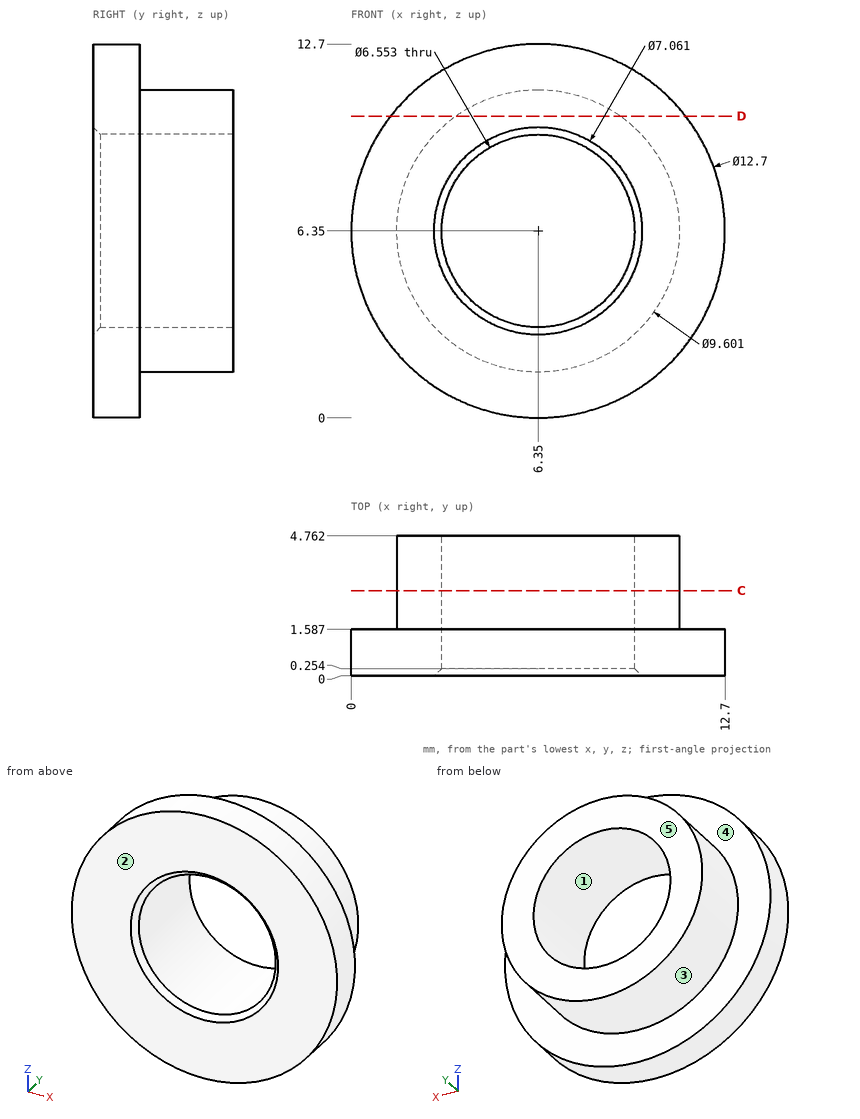
For this review, use the dimensioned drawing (mm, ordinates from the lowest corner) and the shaded views. A direction names the side the tool comes from. Give positions to 0.01 mm unless a question says otherwise; leave off trailing zeros. Loops run counter-clockwise (first coordinate to the right, second up) from the corner with the lowest first, then second, coordinate; pieces in that order, holes last. Notation, with made-up numbers: (67, -39) -> (109, -39) arc R28 cw to (109, -1) -> close; hole circle Ø11 at (0, -34). An arc over 180 degrees is marked (long way). One line per question, with ' | ' between items. Start each with the question number.
(1) Insertion check: P1, Ø1.5, axis at x = 9.5, y = 3, coming from the -Z side; P2, Ø5, axis at x = 6.35, z = 6.35, coming from the -Y side. Each pin has a flat end and moves straight along its axis. Give the tip position at first contact, or say it passes through.
(2) We need section C-C (y = 2.9). State the section outline as (x, z) points.
(3) We need section D-D (z = 10.25). State the section outline as (x, y) points.
(4) For line 1 (X direction, y = 3.25, z = 6.35); line 2 (X direction, y = 1.45, z = 6.35); line 3 (Y direction, x = 9, z = 1.25), list the stretches that pass through material, from the lowest coordinate up.
(5) For the marked faces 4 and 5, list the 3-axis set-ups (+Z, -Z, +X, -X, +Y, -Y) from which the entire face can be reached by the end or side of a thin tool; tool diameter is ignored.
(6) Draft analysis for pull direction Z (two halves, no side actions). For the marked faces 1, 2 and 3, state which applies: +Z half, -Z half, draft (parallel to the pull), parting line (faces both ways), or undercut.
The answers:
1) P1: stops at z = 2.19 | P2: passes through
2) outline: circle Ø9.6 at (6.35, 6.35); hole circle Ø6.55 at (6.35, 6.35)
3) outline: (1.34, 0) -> (11.36, 0) -> (11.36, 1.59) -> (9.15, 1.59) -> (9.15, 4.76) -> (3.55, 4.76) -> (3.55, 1.59) -> (1.34, 1.59) -> close
4) line 1: x = 1.55 to 3.07, 9.63 to 11.15 | line 2: x = 0 to 3.07, 9.63 to 12.7 | line 3: y = 0 to 1.59
5) face 4: +Y | face 5: +Z, -Z, +X, -X, +Y
6) face 1: undercut | face 2: draft | face 3: parting line
